from build123d import *

# Parameters (mm, degrees)
SKETCH1_W               = 64.58
SKETCH1_H               = 35
SKETCH1_R               = 3
BOSS_EXTRUDE1_DEPTH     = 1
CUT_EXTRUDE1_DEPTH      = 37.740904997
CUT_EXTRUDE1_DEPTH_BACK = 37.740904997
SKETCH2_W               = 6
SKETCH2_H               = 17.5
FILLET1_R               = 2
CUT_EXTRUDE2_DEPTH      = 37.740904997
CUT_EXTRUDE2_DEPTH_BACK = 37.740904997
SKETCH3_W               = 35
SKETCH3_H               = 20


with BuildPart() as part:
    # Sketch1 → Boss-Extrude1 (new body)
    with BuildSketch(Plane(origin=(0, 0, 0), x_dir=(1, 0, 0), z_dir=(0, 1, 0))):
        Rectangle(SKETCH1_W, SKETCH1_H)
        with Locations(Location((-25, 0, 0), (0, 0, 270))):
            Circle(SKETCH1_R, mode=Mode.SUBTRACT)
        with Locations(Location((25, 0, 0), (0, 0, 270))):
            Circle(SKETCH1_R, mode=Mode.SUBTRACT)
    extrude(amount=BOSS_EXTRUDE1_DEPTH)

    # Sketch2 → Cut-Extrude1 (cut, two sides: drawn at the far end of the back side and taken through both)
    with BuildSketch(Plane(origin=(0, 1, 0), x_dir=(1, 0, 0), z_dir=(0, 1, 0)).offset(-CUT_EXTRUDE1_DEPTH_BACK)):
        with Locations((-25, 8.75)):
            Rectangle(SKETCH2_W, SKETCH2_H)
        with Locations((25, 8.75)):
            Rectangle(SKETCH2_W, SKETCH2_H)
    extrude(amount=CUT_EXTRUDE1_DEPTH + CUT_EXTRUDE1_DEPTH_BACK, mode=Mode.SUBTRACT)

    # Fillet1
    fillet1_edges = [part.edges().sort_by_distance(p)[0] for p in [
        (22, 0.5, -17.5),
        (-28, 0.5, -17.5),
        (-22, 0.5, -17.5),
        (28, 0.5, -17.5),
    ]]
    fillet(fillet1_edges, radius=FILLET1_R)

    # Sketch3 → Cut-Extrude2 (cut, two sides: drawn at the far end of the back side and taken through both)
    with BuildSketch(Plane.XZ.offset(-CUT_EXTRUDE2_DEPTH_BACK)):
        Rectangle(SKETCH3_W, SKETCH3_H)
    extrude(amount=CUT_EXTRUDE2_DEPTH + CUT_EXTRUDE2_DEPTH_BACK, mode=Mode.SUBTRACT)


solid = part.part
Work out the finished part from the listing and answer in its coordinate system (mm). A direction names the side the tool comes from. Coordinates: 2 decimals unless noted, no trailing zeros. Write each loop counter-clockwise with the first axis right and the second up, starting at its lowest first coordinate (ties: lowest second). Pieces come first, ordered by that corner, then holes. Notation, with made-up numbers: (22.25, 40.5) - (68.25, 40.5) arc R22 cw to (68.25, 57.5) - close; hole circle Ø4 at (89, 46.25). An arc over 180 degrees is marked (long way). One line per question, with ' | ' between items.
1) Consider probe 1 along X at (y, z) = (0.75, -12.5); probe 2 along X at (y, z) = (0.15, -9); probe 3 along Z at (x, y) = (-2, 0.85). Determine where each line is inside the solid, lowest interval first. Write a range as [from, to].
Checks:
probe 1: [-32.29, -28], [-22, 22], [28, 32.29] | probe 2: [-32.29, -28], [-22, -17.5], [17.5, 22], [28, 32.29] | probe 3: [-17.5, -10], [10, 17.5]
2) Find section D-D, the plane z = -8.5. Determine the outline of the cut face in (x, y), and give its area (3 significant figures).
Checks:
outline: (-32.29, 0) - (-28, 0) - (-28, 1) - (-32.29, 1) - close; (-22, 0) - (-17.5, 0) - (-17.5, 1) - (-22, 1) - close; (17.5, 0) - (22, 0) - (22, 1) - (17.5, 1) - close; (28, 0) - (32.29, 0) - (32.29, 1) - (28, 1) - close | area: 17.6 mm2
3) For faces 1 (the face through (0, 1, 11)), 2 (the face through (-28.57, 0.51, -16.9)), determine the directions among +Z, -Z, +X, -X, +Y, -Y from which every point of the face is accessible in a straight line to the end or side of a thin tool.
Checks:
face 1: +Z, -Z, +X, -X, +Y | face 2: -Z, +Y, -Y
4) Find section C-C, the plane y = 0.5. Determine the outline of the cut face in (x, z), and give its area (3 significant figures).
Checks:
outline: (-32.29, -17.5) - (-30, -17.5) arc R2 ccw to (-28, -15.5) - (-28, 0) arc R3 cw to (-22, 0) - (-22, -15.5) arc R2 ccw to (-20, -17.5) - (20, -17.5) arc R2 ccw to (22, -15.5) - (22, 0) arc R3 cw to (28, 0) - (28, -15.5) arc R2 ccw to (30, -17.5) - (32.29, -17.5) - (32.29, 17.5) - (-32.29, 17.5) - close; hole (-17.5, -10) - (17.5, -10) - (17.5, 10) - (-17.5, 10) - close | area: 1,320 mm2
5) Find section B-B, the plane x = 9.5. Determine the outline of the cut face in (y, z), and give its area (3 significant figures).
Checks:
outline: (0, -17.5) - (1, -17.5) - (1, -10) - (0, -10) - close; (0, 10) - (1, 10) - (1, 17.5) - (0, 17.5) - close | area: 15.0 mm2
6) The mould has two halves that part along X. Classify faces 3 (the face through (0, 0, 11)), 4 (the face through (24.9, 0.5, 3)): +X half, -X half, draft (parallel to the pull), parting line (faces both ways), or undercut.
Checks:
face 3: draft | face 4: undercut
7) Find section A-A, the plane z = 4.5. Determine the outline of the cut face in (x, y).
Checks:
outline: (-32.29, 0) - (-17.5, 0) - (-17.5, 1) - (-32.29, 1) - close; (17.5, 0) - (32.29, 0) - (32.29, 1) - (17.5, 1) - close
8) A flat-ended cylindrical pin translates along its axis: P1, Ø12, axis at x = -10, z = -2.5, coming from the -Y side. Find the tip coordinate at first contact, or state that the pin passes through.
Checks:
P1: through
